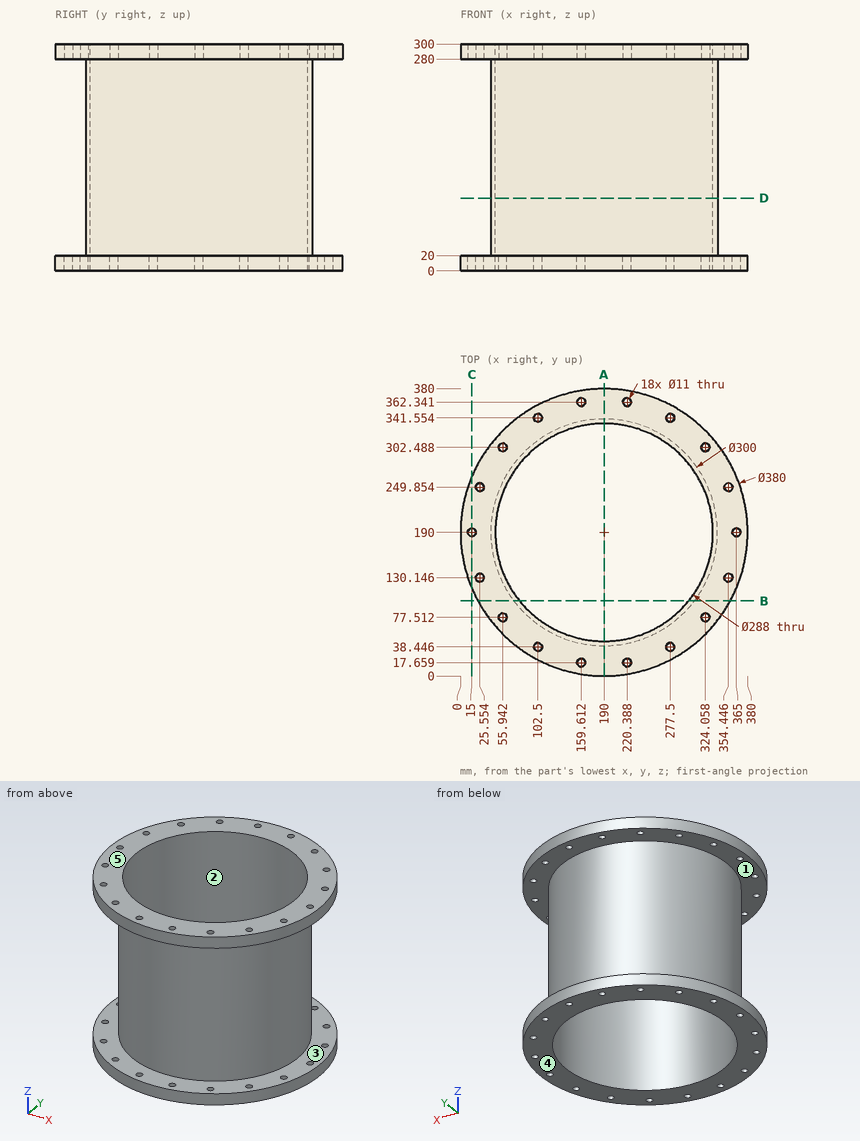
Input: dimensioned drawing with shaded views. Units: mm. Origin: part minimum x, y, z. A direction names the side the tool comes from. Round coordinates to 2 decimals unless told otherwise and drop trailing zeros. Order: outer loops, then holes, each group sorted by start corner. A loop starts at its lowest first (then second) coordinate and runs counter-clockwise, first axis right, second up. Notation, with made-up numbers: (24.25, 89) -> (74.25, 89) arc R17 cw to (74.25, 106) -> close; hole circle Ø4 at (32.5, 62.5). An arc over 180 degrees is marked (long way). Put each result on its own line as item: value. Start each with the question number.
Q1. Line query: probe 1 along Z at (x, y) = (229, 19); probe 2 along X at (y, z) = (190, 159.5); probe 3 along Y at (x, z) = (129, 278) (1 decimal). Output: solid intervals per line, ascending.
Q2. First-contact query: pin 1 (9 mm diameter, centred on x = 220.39, y = 362.34, fed in from +Z); pin 2 (8 mm diameter, centred on x = 271.5, z = 42.5, fed in from +Y); pin 3 (2 mm diameter, centred on x = 254, z = 64.5, fed in from +Y); pin 4 (8 mm diameter, centred on x = 80, z = 103, fed in from -Y). Flat tips, straight axial feed; report the tip coordinate or a pass-through.
Q3. Section D-D on z = 96. Return the cut outline in (x, y), and give its area (3 significant figures).
Q4. Section B-B on y = 99.5. Return the cut outline in (x, z).
Q5. Section C-C on x = 15. Return the cut outline in (y, z).
Q6. Section A-A on x = 190. Return the cut outline in (y, z), and give its area (3 significant figures).
Q7. Pull-direction query (Z, two-part tool) for the marked faces 3, 4 and 5; classes: +Z half, -Z half, draft (parallel to the pull), parting line (faces both ways), or undercut.
Q8. Reachability of the marked faces 1 and 2 from +Z, -Z, +X, -X, +Y, -Y: full face, straight path, thin tool, end or side. Return the list, or none.
Ans:
1. probe 1: z = 0 to 20, 280 to 300
1. probe 2: x = 40 to 46, 334 to 340
1. probe 3: y = 53 to 59.6, 320.4 to 327
2. pin 1: passes through
2. pin 2: stops at y = 318.43
2. pin 3: stops at y = 326.13
2. pin 4: stops at y = 83.87
3. outline: circle Ø300 at (190, 190); hole circle Ø288 at (190, 190)
3. area: 5,540 mm2
4. outline: (22.94, 0) -> (77.99, 0) -> (77.99, 300) -> (22.94, 300) -> (22.94, 280) -> (70.38, 280) -> (70.38, 20) -> (22.94, 20) -> close; (302.01, 0) -> (357.06, 0) -> (357.06, 20) -> (309.62, 20) -> (309.62, 280) -> (357.06, 280) -> (357.06, 300) -> (302.01, 300) -> close
5. outline: (116.01, 0) -> (184.5, 0) -> (184.5, 20) -> (116.01, 20) -> close; (116.01, 280) -> (184.5, 280) -> (184.5, 300) -> (116.01, 300) -> close; (195.5, 0) -> (263.99, 0) -> (263.99, 20) -> (195.5, 20) -> close; (195.5, 280) -> (263.99, 280) -> (263.99, 300) -> (195.5, 300) -> close
6. outline: (0, 0) -> (46, 0) -> (46, 300) -> (0, 300) -> (0, 280) -> (40, 280) -> (40, 20) -> (0, 20) -> close; (334, 0) -> (380, 0) -> (380, 20) -> (340, 20) -> (340, 280) -> (380, 280) -> (380, 300) -> (334, 300) -> close
6. area: 6,800 mm2
7. face 3: undercut
7. face 4: -Z half
7. face 5: +Z half
8. face 1: none
8. face 2: +Z, -Z
